from build123d import *

# Parameters (mm, degrees)
SKETCH1_R           = 18.5
BOSS_EXTRUDE1_DEPTH = 27
SKETCH2_R           = 1.5
CUT_EXTRUDE1_DEPTH  = 5
CIRPATTERN1_COUNT   = 3
SKETCH3_R           = 6
BOSS_EXTRUDE2_DEPTH = 6
SKETCH4_R           = 3
BOSS_EXTRUDE3_DEPTH = 15
CUT_EXTRUDE2_DEPTH  = 12
SKETCH6_R           = 13.8
BOSS_EXTRUDE4_DEPTH = 46.4
SKETCH7_R           = 3
BOSS_EXTRUDE5_DEPTH = 9.5


with BuildPart() as part:
    # Sketch1 → Boss-Extrude1 (new body)
    with BuildSketch(Plane(origin=(0, 0, 0), x_dir=(1, 0, 0), z_dir=(0, 1, 0))):
        Circle(SKETCH1_R)
    extrude(amount=BOSS_EXTRUDE1_DEPTH)

    # Sketch2 → Cut-Extrude1 (cut)
    with BuildSketch(Plane(origin=(0, 27, 0), x_dir=(1, 0, 0), z_dir=(0, 1, 0))):
        with Locations((0, 15.5)):
            Circle(SKETCH2_R)
        with Locations((-7.75, 13.423393759)):
            Circle(SKETCH2_R)
    cut_extrude1 = extrude(amount=-CUT_EXTRUDE1_DEPTH, mode=Mode.SUBTRACT)

    # CirPattern1: Cut-Extrude1 ×3 about axis
    cirpattern1_axis = Axis((0, 0, 0), (0, 1, 0))
    for i in range(1, CIRPATTERN1_COUNT):
        add(cut_extrude1.rotate(cirpattern1_axis, i * 360 / CIRPATTERN1_COUNT), mode=Mode.SUBTRACT)

    # Sketch3 → Boss-Extrude2 (add)
    with BuildSketch(Plane(origin=(0, 27, 0), x_dir=(1, 0, 0), z_dir=(0, 1, 0))):
        with Locations((0, -7)):
            Circle(SKETCH3_R)
    extrude(amount=BOSS_EXTRUDE2_DEPTH)

    # Sketch4 → Boss-Extrude3 (add)
    with BuildSketch(Plane(origin=(0, 33, 0), x_dir=(1, 0, 0), z_dir=(0, 1, 0))):
        with Locations((0, -7)):
            Circle(SKETCH4_R)
    extrude(amount=BOSS_EXTRUDE3_DEPTH)

    # Sketch5 → Cut-Extrude2 (cut)
    with BuildSketch(Plane(origin=(0, 48, 0), x_dir=(1, 0, 0), z_dir=(0, 1, 0))):
        with BuildLine():
            Line((-1.658312395, -4.5), (1.658312395, -4.5))
            ThreePointArc((1.658312395, -4.5), (0, -4), (-1.658312395, -4.5))
        make_face()
    extrude(amount=-CUT_EXTRUDE2_DEPTH, mode=Mode.SUBTRACT)

    # Sketch6 → Boss-Extrude4 (add)
    with BuildSketch(Plane.XZ):
        Circle(SKETCH6_R)
    extrude(amount=BOSS_EXTRUDE4_DEPTH)

    # Sketch7 → Boss-Extrude5 (add)
    with BuildSketch(Plane.XZ.offset(46.4)):
        Circle(SKETCH7_R)
    extrude(amount=BOSS_EXTRUDE5_DEPTH)


solid = part.part
Here's how the part is built. I have some questions about the finished solid (model axes, mm). A direction names the side the tool comes from. Give positions to 0.01 mm unless a question says otherwise; leave off trailing zeros. Order: outer loops, then holes, each group sorted by start corner. A loop starts at its lowest first (then second) coordinate and runs counter-clockwise, first axis right, second up. Notation, with made-up numbers: M 50,-14 L 71,-14 A24 cw 71,-3 Z; hole C 71.25,32 d3. An arc over 180 degrees is marked long. Answer as a JSON object with one key per item and string values. Group by question number.
1) Suppose I cut it at D-D, the plane z = -6. Write out the boundary of the cut face in (x, y).
2) I'm going to push flat-ended pins straight in: pin 1 Ø12 at (x, y) = (-3.5, -23) entering from +Z; pin 2 Ø10 at (x, z) = (5.5, 0) entering from +Y; pin 3 Ø1.5 at (x, z) = (-13, 7) entering from +Y. Where does each tip first touch, or does it pass through?
3) On a 3-axis mill with a long thin cutter (end or side, diameter ignored), from which of +Z, -Z, +X, -X, +Y, -Y can I reach the whole of each face in a straight line? I mean faces 1 (the cylindrical face through (-4.01, 13.31, 18.06)), 2 (the cylindrical face through (12.318, 24.535, 6.736)), 3 (the cylindrical face through (-3, -51, 0)). Say none if no direction works.
4) Suppose I cut it at C-C, the plane y = -12.5. Write out the boundary of the cut face in (x, z), plus the area to 3 significant figures.
5) Please list where these lines run through material, in increasing order: L1, parallel to Z at x = 0, y = 24.8; L2, parallel to Y at x = 8.5, z = -15.5; L3, parallel to Y at x = 7.5, z = 4.5. Write a range as [from, to].
6) Suppose I cut it at B-B, the plane z = 0. Write out the boundary of the cut face in (x, y), plus the area to 3 significant figures.
7) We'd pull the mould along Z, two halves only. Please class faces 4 (the cylindrical face through (-6, 30, 7)), 5 (the flat face through (16, 22, 0)), 6 (the flat face through (0, 48, 7)): pulls with the +Z half, pulls with the -Z half, needs draft (parallel to the pull), parting line crosses it, or undercut.
8) Suppose I cut it at A-A, the plane x = 0. Write out the boundary of the cut face in (y, z), plus the area to 3 significant figures.
Results found:
{
 "1": {"outline": "M -17.5,0 L -12.43,0 L -12.43,-46.4 L 12.43,-46.4 L 12.43,0 L 17.5,0 L 17.5,27 L -17.5,27 Z"},
 "2": {"pin 1": "z = 13.8", "pin 2": "y = 33", "pin 3": "y = 27"},
 "3": {"face 1": "+Y, -Y", "face 2": "+Y", "face 3": "-Y"},
 "4": {"outline": "C 0,0 d27.6", "area": "598 mm²"},
 "5": {"L1": "[-18.5, -17], [-14, 18.5]", "L2": "[0, 27]", "L3": "[-46.4, 27]"},
 "6": {"outline": "M -18.5,0 L -13.8,0 L -13.8,-46.4 L -3,-46.4 L -3,-55.9 L 3,-55.9 L 3,-46.4 L 13.8,-46.4 L 13.8,0 L 18.5,0 L 18.5,27 L 17,27 L 17,22 L 14,22 L 14,27 L -18.5,27 Z", "area": "2,320 mm²"},
 "7": {"face 4": "parting line crosses it", "face 5": "undercut", "face 6": "needs draft"},
 "8": {"outline": "M -55.9,-3 L -46.4,-3 L -46.4,-13.8 L 0,-13.8 L 0,-18.5 L 27,-18.5 L 27,-17 L 22,-17 L 22,-14 L 27,-14 L 27,1 L 33,1 L 33,4 L 36,4 L 36,4.5 L 48,4.5 L 48,10 L 33,10 L 33,13 L 27,13 L 27,18.5 L 0,18.5 L 0,13.8 L -46.4,13.8 L -46.4,3 L -55.9,3 Z", "area": "2,480 mm²"}
}
